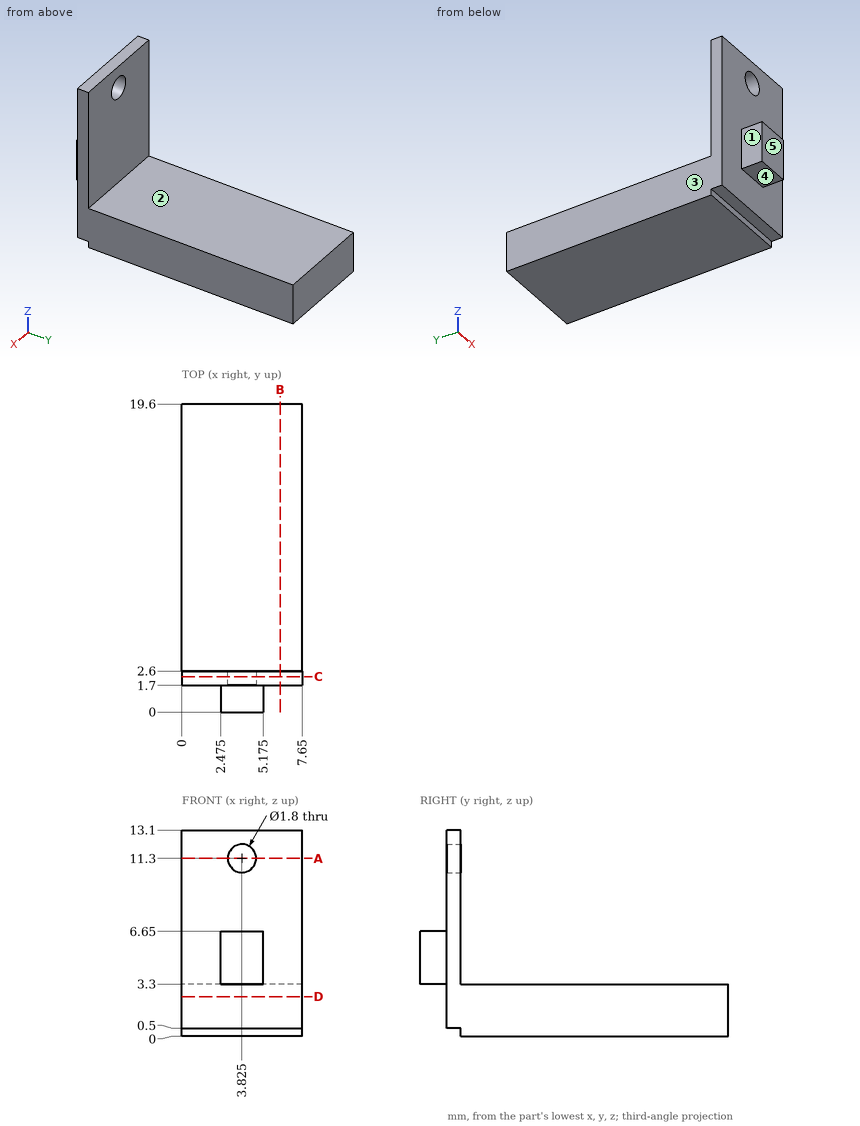
Source: three-view drawing plus pictorial views. Frame: mm from the lowest corner of the part. A direction names the side the tool comes from. Give positions to 0.01 mm unless a question says otherwise; leave off trailing zeros. Order: outer loops, then holes, each group sorted by start corner. A loop starts at its lowest first (then second) coordinate and runs counter-clockwise, first axis right, second up. Notation, with made-up numbers: (-26, 23.25) - (-15, 23.25) arc R30 ccw to (-15, 58.25) - close; hole circle Ø1 at (88.25, -15). An arc over 180 degrees is marked (long way). Answer as a JSON object with one key per item and string values. Group by question number.
Q1. Line query: probe 1 along Y at (x, z) = (2, 6.5); probe 2 along Z at (x, y) = (4, 1); probe 3 along Z at (x, y) = (6.75, 3.5). Output: solid intervals per line, ascending.
Q2. Cut plane B-B, the plane x = 6.25. Output: boundary loops of the cut face in (y, z), then the cut area to 3 significant figures.
Q3. Cut plane D-D, the plane z = 2.5. Output: boundary loops of the cut face in (x, y), then the cut area to 3 significant figures.
Q4. First-contact query: pin 1 Ø4 at (x, y) = (3.5, 5) entering from +Z; pin 2 Ø1.9 at (y, z) = (0.5, 5) entering from +X (3 decimals); pin 3 Ø4 at (x, z) = (7, 8.5) entering from +Y; pin 4 Ø0.8 at (x, y) = (3.5, 1.5) entering from +Z. Flat tips, straight axial feed; report the tip coordinate or a pass-through.
Q5. Cut plane C-C, the plane y = 2.25. Output: boundary loops of the cut face in (x, z) (3 decimals).
Q6. Set-up query: the marked faces 1, 2, 3, 4 and 5. Return all of +Z, -Z, +X, -X, +Y, -Y with unobstructed straight access to the full face (end or side cutting, diameter ignored); none if empty.
Q7. Cut plane A-A, the plane z = 11.3. Output: boundary loops of the cut face in (x, y) (3 decimals), then the cut area to 4 significant figures.
Results:
{
 "1": {"probe 1": "1.7 to 2.6", "probe 2": "3.3 to 6.65", "probe 3": "0 to 3.3"},
 "2": {"outline": "(1.7, 0.5) - (2.6, 0.5) - (2.6, 0) - (19.6, 0) - (19.6, 3.3) - (2.6, 3.3) - (2.6, 13.1) - (1.7, 13.1) - close", "area": "67.4 mm^2"},
 "3": {"outline": "(0, 1.7) - (7.65, 1.7) - (7.65, 19.6) - (0, 19.6) - close", "area": "137 mm^2"},
 "4": {"pin 1": "z = 3.3", "pin 2": "x = 5.175", "pin 3": "y = 2.6", "pin 4": "z = 13.1"},
 "5": {"outline": "(0, 0.5) - (7.65, 0.5) - (7.65, 13.1) - (0, 13.1) - close; hole circle Ø1.8 at (3.825, 11.3)"},
 "6": {"face 1": "+Z, -Z, -X, -Y", "face 2": "+Z, +X, -X, +Y", "face 3": "+Z, -Z, -X, +Y, -Y", "face 4": "-Z, +X, -X, -Y", "face 5": "+Z, -Z, +X, -X, -Y"},
 "7": {"outline": "(0, 1.7) - (2.925, 1.7) - (2.925, 2.6) - (0, 2.6) - close; (4.725, 1.7) - (7.65, 1.7) - (7.65, 2.6) - (4.725, 2.6) - close", "area": "5.265 mm^2"}
}
